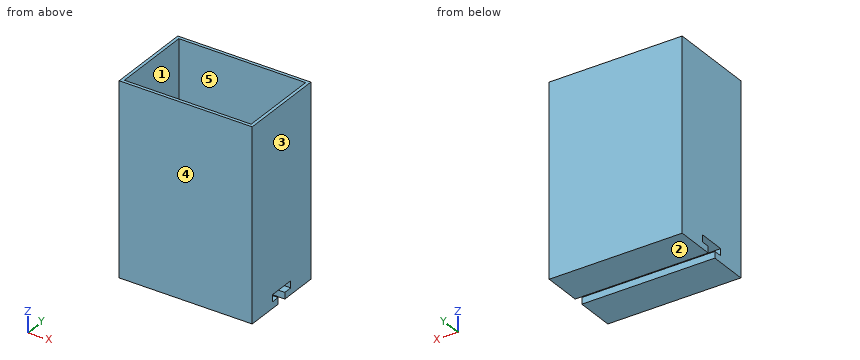
```python
from build123d import *

# Parameters (mm, degrees)
F0_W     = 67.945
F0_H     = 44.45
F1_DEPTH = 1.5875
F2_W     = 67.945
F2_H     = 44.45
F2_W_2   = 64.77
F2_H_2   = 41.275
F3_DEPTH = 88.9
F4_W     = 67.945
F4_H     = 15.24
F5_DEPTH = 6.858
F6_W     = 67.945
F6_H     = 4.445
F7_DEPTH = 3.302


with BuildPart() as f1:
    # F0 (on Top) → F1 (new body)
    with BuildSketch(Plane.XY):
        Rectangle(F0_W, F0_H)
    extrude(amount=F1_DEPTH)

    # F2 (on face) → F3 (join)
    with BuildSketch(Plane.XY.offset(1.5875)):
        Rectangle(F2_W, F2_H)
        Rectangle(F2_W_2, F2_H_2, mode=Mode.SUBTRACT)
    extrude(amount=F3_DEPTH)

    # F4 (on face) → F5 (join)
    with BuildSketch(Plane(origin=(0, 0, 0), x_dir=(1, 0, 0), z_dir=(0, 0, -1))):
        with Locations((0, 14.605)):
            Rectangle(F4_W, F4_H)
        with Locations((0, -14.605)):
            Rectangle(F4_W, F4_H)
    extrude(amount=F5_DEPTH)

    # F6 (on face) → F7 (join)
    with BuildSketch(Plane(origin=(0, 0, -6.858), x_dir=(1, 0, 0), z_dir=(0, 0, -1))):
        with Locations((0, 4.7625)):
            Rectangle(F6_W, F6_H)
        with Locations((0, -4.7625)):
            Rectangle(F6_W, F6_H)
    extrude(amount=-F7_DEPTH)


solid = f1.part
```
Design review of the part built by this model. Coordinates are the model's own, in mm. Face numbers are marked on the shaded views. A direction names the side the tool comes from. Round coordinates to 2 decimals unless told otherwise and drop trailing zeros. Write each loop counter-clockwise with the first axis right and the second up, starting at its lowest first coordinate (ties: lowest second). Pieces come first, ordered by that corner, then holes. Notation, with made-up numbers: (-15, -27.5) -> (18, -27.5) arc R19 ccw to (18, 7.5) -> close; hole circle Ø3 at (35, -22.75). An arc over 180 degrees is marked (long way). Write item = value, one per line. Start each with the question number.
1) Clearance check with flat-ended pins moving along their axes: pin 1 (10 mm diameter, centred on x = -8.5, y = 7.5, fed in from +Z); pin 2 (1 mm diameter, centred on x = 17.5, y = 1, fed in from -Z). State where each tip first meets the part, or that it passes through.
2) Tool access review of the marked faces 1 and 2: name each direction out of +Z, -Z, +X, -X, +Y, -Y from which nothing blocks a thin tool from reaching the whole face with its end or side.
3) Take a section at B-B, the plane y = -10.5. State the section outline as (x, z) points (1 decimal), plus the area to 3 significant figures.
4) Mouldability with a two-part tool opening along Y and no side actions: class the marked faces 3, 4 and 5 as +Y half, -Y half, draft (parallel to the pull), parting line (faces both ways), or undercut.
5) Wall thickness on probe 1 along Y at (x, z) = (10, 77) (1 decimal); probe 2 along X at (y, z) = (8.5, 87.5) (1 decimal); probe 3 along Z at (x, y) = (-3, -6): over which ranges is each line inside the solid? List them lowest first. Write a range as from..to.
6) Take a section at A-A, the plane z = 62.5. State the section outline as (x, y) points (1 decimal), plus the area to 3 significant figures.
7) Take a section at C-C, the plane x = 12. State the section outline as (y, z) points (1 decimal), plus the area to 3 significant figures.
Results list:
q1.pin_1 = 1.59
q1.pin_2 = 0
q2.face_1 = +Z
q2.face_2 = -Z, +X, -X, +Y, -Y
q3.outline = (-34, -6.9) -> (34, -6.9) -> (34, 90.5) -> (32.4, 90.5) -> (32.4, 1.6) -> (-32.4, 1.6) -> (-32.4, 90.5) -> (-34, 90.5) -> close
q3.area = 856 mm²
q4.face_3 = draft
q4.face_4 = -Y half
q4.face_5 = undercut
q5.probe_1 = -22.2..-20.6, 20.6..22.2
q5.probe_2 = -34..-32.4, 32.4..34
q5.probe_3 = -6.86..-3.56, 0..1.59
q6.outline = (-34, -22.2) -> (34, -22.2) -> (34, 22.2) -> (-34, 22.2) -> close; hole (-32.4, -20.6) -> (32.4, -20.6) -> (32.4, 20.6) -> (-32.4, 20.6) -> close
q6.area = 347 mm²
q7.outline = (-22.2, -6.9) -> (-2.5, -6.9) -> (-2.5, -3.6) -> (-7, -3.6) -> (-7, 0) -> (7, 0) -> (7, -3.6) -> (2.5, -3.6) -> (2.5, -6.9) -> (22.2, -6.9) -> (22.2, 90.5) -> (20.6, 90.5) -> (20.6, 1.6) -> (-20.6, 1.6) -> (-20.6, 90.5) -> (-22.2, 90.5) -> close
q7.area = 591 mm²
